Geometry: final body of the model. Coordinates: model frame, mm. A direction names the side the tool comes from. Give positions to 0.01 mm unless a question says otherwise; leave off trailing zeros. Loops run counter-clockwise (first coordinate to the right, second up) from the corner with the lowest first, then second, coordinate; pieces in that order, holes last. Notation, with made-up numbers: (-26.5, 2.5) - (28.5, 2.5) arc R27 cw to (28.5, 24.5) - close; hole circle Ø9 at (-32.75, -12). An arc over 180 degrees is marked (long way). Answer in a Markdown table with one row per item.
Autodesk Inventor part; units mm, degrees
ref_plane "YZ Plane" through (0, 0, 0) normal (1, 0, 0) x (0, 1, 0)
ref_plane "XZ Plane" through (0, 0, 0) normal (0, 1, 0) x (-1, 0, 0)
ref_plane "XY Plane" through (0, 0, 0) normal (0, 0, 1) x (1, 0, 0)
sketch "Náčrt1" plane through (0, 0, 0) normal (0, 1, 0) x (-1, 0, 0)
  circle A0 centre (0, 0) radius 16.1
  circle A1 centre (0, 0) radius 14.175
  circle A2 centre (0, 0) radius 10
  circle A3 centre (0, 0) radius 8.5
  dimension "d0" = 32.2
  dimension "d1" = 28.35
  dimension "d2" = 20
  dimension "d3" = 1.5
extrude "Vysunutí1" add sketch "Náčrt1" along normal blind 1 contours A0
extrude "Vysunutí2" add sketch "Náčrt1" along normal blind 5 contours A1
extrude "Vysunutí3" add sketch "Náčrt1" along normal blind 28 contours A2 | A3
extrude "Vysunutí4" cut sketch "Náčrt1" along normal blind 26.5 contours A3
fillet "Zaoblení1" radius 2.5 1 edges at (8.5, 26.5, 0)
chamfer "Zkosení1" distance 2 angle 45 1 edges at (8.5, 0, 0)
properties part number "D28 - Forma"
Q1. Cut plane C-C (y = 19.5). Output: boundary loops of the cut face in (x, z).
Check values:
| item | result |
|---|---|
| outline | circle Ø20 at (0, 0); hole circle Ø17 at (0, 0) |
Q2. Cut plane D-D (x = 12). Output: boundary loops of the cut face in (y, z).
Check values:
| item | result |
|---|---|
| outline | (0, -10.73) - (1, -10.73) - (1, -7.55) - (5, -7.55) - (5, 7.55) - (1, 7.55) - (1, 10.73) - (0, 10.73) - close |
Q3. Material intervals for line 1 along Z through (x, y) = (0, 19.5); line 2 along Y through (x, z) = (-3.5, 13.5); line 3 along Y through (x, z) = (-6, 13), sorted ascending.
Check values:
| item | result |
|---|---|
| line 1 | -10 to -8.5, 8.5 to 10 |
| line 2 | 0 to 5 |
| line 3 | 0 to 1 |
Q4. Cut plane A-A (x = 0). Output: boundary loops of the cut face in (y, z) (3 decimals).
Check values:
| item | result |
|---|---|
| outline | (0, -16.1) - (1, -16.1) - (1, -14.175) - (5, -14.175) - (5, -10) - (28, -10) - (28, 10) - (5, 10) - (5, 14.175) - (1, 14.175) - (1, 16.1) - (0, 16.1) - (0, 10.5) - (2, 8.5) - (24, 8.5) arc R2.5 cw to (26.5, 6) - (26.5, -6) arc R2.5 cw to (24, -8.5) - (2, -8.5) - (0, -10.5) - close |
Q5. Draft query along X for faces 4 (the cylindrical face through (-7.62, 2.972, -11.952)), 5 (the conical face through (1.87, 1.875, 8.42)), 6 (the flat face through (0, 26.5, 0)), 7 (the flat face through (-8, 1, -12)). Return one class per face: pulls with the +X half, pulls with the -X half, needs draft (parallel to the pull), parting line crosses it, or undercut.
Check values:
| item | result |
|---|---|
| face 4 | parting line crosses it |
| face 5 | undercut |
| face 6 | undercut |
| face 7 | needs draft |
Q6. First-contact query: pin 1 (5 mm diameter, centred on x = 7.5, y = 18, fed in from -Z); pin 2 (6 mm diameter, centred on x = 0, y = 5.5, fed in from +Z) (3 decimals); pin 3 (8 mm diameter, centred on y = 11, z = 10.5, fed in from +X). Flat tips, straight axial feed; report the tip coordinate or a pass-through.
Check values:
| item | result |
|---|---|
| pin 1 | z = -8.66 |
| pin 2 | z = 14.175 |
| pin 3 | x = 7.6 |
Q7. Cut plane B-B (z = 0). Output: boundary loops of the cut face in (x, y) (3 decimals).
Check values:
| item | result |
|---|---|
| outline | (-16.1, 0) - (-10.5, 0) - (-8.5, 2) - (-8.5, 24) arc R2.5 cw to (-6, 26.5) - (6, 26.5) arc R2.5 cw to (8.5, 24) - (8.5, 2) - (10.5, 0) - (16.1, 0) - (16.1, 1) - (14.175, 1) - (14.175, 5) - (10, 5) - (10, 28) - (-10, 28) - (-10, 5) - (-14.175, 5) - (-14.175, 1) - (-16.1, 1) - close |
Q8. Reachability of faces 1 (the cylindrical face through (-4.57, 12.846, -7.167)), 2 (the flat face through (0, 28, 0)), 3 (the cylindrical face through (2.17, 16.34, 9.76)) from +Z, -Z, +X, -X, +Y, -Y: full face, straight path, thin tool, end or side. Return the list, or none.
Check values:
| item | result |
|---|---|
| face 1 | -Y |
| face 2 | +Z, -Z, +X, -X, +Y |
| face 3 | +Y |
